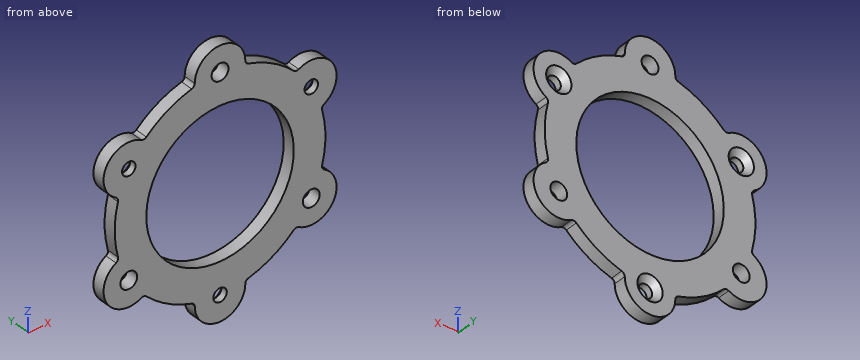
from build123d import *

# Parameters (mm, degrees)
SKETCH1_R                     = 8.75
SKETCH1_R_2                   = 1
BOSS_EXTRUDE1_DEPTH           = 1.5
CSK_FOR_M3_SFHCS1_D           = 1.6
CSK_FOR_M3_SFHCS1_DEPTH       = 7.5
CSK_FOR_M3_SFHCS1_CSINK_D     = 3
CSK_FOR_M3_SFHCS1_CSINK_ANGLE = 90
CSK_FOR_M3_SFHCS1_TIP         = 0.480688495
FILLET1_R                     = 0.5


with BuildPart() as part:
    # Sketch1 → Boss-Extrude1 (new body)
    with BuildSketch(Plane(origin=(0, 0, 0), x_dir=(1, 0, 0), z_dir=(0, 1, 0))):
        with BuildLine():
            Line((-3, -12.1346611), (-3, -12.5))
            ThreePointArc((-3, -12.5), (0, -15.5), (3, -12.5))
            Line((3, -12.5), (3, -12.1346611))
            ThreePointArc((3, -12.1346611), (6.25, -10.825317547), (9.008924778, -8.665406761))
            Line((9.008924778, -8.665406761), (9.325317547, -8.848076211))
            ThreePointArc((9.325317547, -8.848076211), (13.423393759, -7.75), (12.325317547, -3.651923789))
            Line((12.325317547, -3.651923789), (12.008924778, -3.469254338))
            ThreePointArc((12.008924778, -3.469254338), (12.5, 0), (12.008924778, 3.469254338))
            Line((12.008924778, 3.469254338), (12.325317547, 3.651923789))
            ThreePointArc((12.325317547, 3.651923789), (13.423393759, 7.75), (9.325317547, 8.848076211))
            Line((9.325317547, 8.848076211), (9.008924778, 8.665406761))
            ThreePointArc((9.008924778, 8.665406761), (6.25, 10.825317547), (3, 12.1346611))
            Line((3, 12.1346611), (3, 12.5))
            ThreePointArc((3, 12.5), (0, 15.5), (-3, 12.5))
            Line((-3, 12.5), (-3, 12.1346611))
            ThreePointArc((-3, 12.1346611), (-6.25, 10.825317547), (-9.008924778, 8.665406761))
            Line((-9.008924778, 8.665406761), (-9.325317547, 8.848076211))
            ThreePointArc((-9.325317547, 8.848076211), (-13.423393759, 7.75), (-12.325317547, 3.651923789))
            Line((-12.325317547, 3.651923789), (-12.008924778, 3.469254338))
            ThreePointArc((-12.008924778, 3.469254338), (-12.5, 0), (-12.008924778, -3.469254338))
            Line((-12.008924778, -3.469254338), (-12.325317547, -3.651923789))
            ThreePointArc((-12.325317547, -3.651923789), (-13.423393759, -7.75), (-9.325317547, -8.848076211))
            Line((-9.325317547, -8.848076211), (-9.008924778, -8.665406761))
            ThreePointArc((-9.008924778, -8.665406761), (-6.25, -10.825317547), (-3, -12.1346611))
        make_face()
        with Locations(Location((0, 0, 0), (0, 0, 270))):
            Circle(SKETCH1_R, mode=Mode.SUBTRACT)
        with Locations(Location((-10.825317547, 6.25, 0), (0, 0, 270))):
            Circle(SKETCH1_R_2, mode=Mode.SUBTRACT)
        with Locations(Location((10.825317547, 6.25, 0), (0, 0, 270))):
            Circle(SKETCH1_R_2, mode=Mode.SUBTRACT)
        with Locations(Location((0, -12.5, 0), (0, 0, 270))):
            Circle(SKETCH1_R_2, mode=Mode.SUBTRACT)
    extrude(amount=BOSS_EXTRUDE1_DEPTH)

    # CSK for M3 SFHCS1
    with Locations(Plane(origin=(-10.825317547, 1.5, 6.25), x_dir=(0, 0, 1), z_dir=(0, 1, 0))):
        with Locations((0, 0), (-18.75, 10.825317547), (0, 21.650635094)):
            CounterSinkHole(CSK_FOR_M3_SFHCS1_D / 2, CSK_FOR_M3_SFHCS1_CSINK_D / 2, depth=CSK_FOR_M3_SFHCS1_DEPTH, counter_sink_angle=CSK_FOR_M3_SFHCS1_CSINK_ANGLE)
            with Locations((0, 0, -(CSK_FOR_M3_SFHCS1_DEPTH + CSK_FOR_M3_SFHCS1_TIP / 2))):  # 118° drill point
                Cone(0, CSK_FOR_M3_SFHCS1_D / 2, CSK_FOR_M3_SFHCS1_TIP, mode=Mode.SUBTRACT)

    # Fillet1
    fillet1_edges = [part.edges().sort_by_distance(p)[0] for p in [
        (-3, 0.75, 12.1346611),
        (3, 0.75, 12.1346611),
        (9.008924778, 0.75, 8.665406761),
        (12.008924778, 0.75, 3.469254338),
        (12.008924778, 0.75, -3.469254338),
        (9.008924778, 0.75, -8.665406761),
        (3, 0.75, -12.1346611),
        (-3, 0.75, -12.1346611),
        (-9.008924778, 0.75, -8.665406761),
        (-12.008924778, 0.75, -3.469254338),
        (-12.008924778, 0.75, 3.469254338),
        (-9.008924778, 0.75, 8.665406761),
    ]]
    fillet(fillet1_edges, radius=FILLET1_R)


solid = part.part
The model under review builds one solid part; all positions refer to its coordinate system, in mm. Round coordinates to 2 decimals unless told otherwise and drop trailing zeros. Order: outer loops, then holes, each group sorted by start corner. A loop starts at its lowest first (then second) coordinate and runs counter-clockwise, first axis right, second up. Notation, with made-up numbers: (43.25, -31.75) -> (64.25, -31.75) arc R31 cw to (64.25, 6.25) -> close; hole circle Ø4 at (-28, 63.5). An arc over 180 degrees is marked (long way). Return JSON: item names as keys, results as strings.
1. Take a section at A-A (x = 0). Write out the cut boundary in (y, z).
Answer block:
{"outline": "(0, -15.5) -> (1.5, -15.5) -> (1.5, -14) -> (0.8, -13.3) -> (0, -13.3) -> close; (0, -11.7) -> (0.8, -11.7) -> (1.5, -11) -> (1.5, -8.75) -> (0, -8.75) -> close; (0, 8.75) -> (1.5, 8.75) -> (1.5, 11.5) -> (0, 11.5) -> close; (0, 13.5) -> (1.5, 13.5) -> (1.5, 15.5) -> (0, 15.5) -> close"}
2. Take a section at D-D (y = 0.35). State how many separate pieces and enclosed holes the cut face has, then the cut area to 3 significant figures.
Answer block:
{"separate pieces": "1", "enclosed holes": "7", "area": "324 mm²"}
3. For L1, parallel to X at y = 0.9, z = 0; L2, parallel to Z at x = -0.5, y = 0.6; L3, parallel to X at y = 0.9, z = -6.25, list the stretches that pass through material, from the lowest coordinate up. Write a range as [from, to].
Answer block:
{"L1": "x = [-12.5, -8.75], [8.75, 12.5]", "L2": "z = [-15.46, -13.12], [-11.88, -8.74], [8.74, 11.63], [13.37, 15.46]", "L3": "x = [-13.83, -11.83], [-9.83, -6.12], [6.12, 9.83], [11.83, 13.83]"}
4. Take a section at B-B (z = 0). Write out the cut boundary in (x, y).
Answer block:
{"outline": "(-12.5, 0) -> (-8.75, 0) -> (-8.75, 1.5) -> (-12.5, 1.5) -> close; (8.75, 0) -> (12.5, 0) -> (12.5, 1.5) -> (8.75, 1.5) -> close"}
5. Take a section at C-C (z = 6.25). Write out the cut boundary in (x, y).
Answer block:
{"outline": "(-13.83, 0) -> (-11.63, 0) -> (-11.63, 0.8) -> (-12.33, 1.5) -> (-13.83, 1.5) -> close; (-10.03, 0) -> (-6.12, 0) -> (-6.12, 1.5) -> (-9.33, 1.5) -> (-10.03, 0.8) -> close; (6.12, 0) -> (10.03, 0) -> (10.03, 0.8) -> (9.33, 1.5) -> (6.12, 1.5) -> close; (11.63, 0) -> (13.83, 0) -> (13.83, 1.5) -> (12.33, 1.5) -> (11.63, 0.8) -> close"}
